CAD build for the part. Positions are in the model's coordinates, mm. Coordinates: 2 decimals unless noted, no trailing zeros. Loops run counter-clockwise (first coordinate to the right, second up) from the corner with the lowest first, then second, coordinate; pieces in that order, holes last. Notation, with made-up numbers: (-30.75, 18) -> (-22.75, 18) arc R8 cw to (-22.75, 31) -> close; hole circle Ø4 at (8.5, -4). An arc over 180 degrees is marked (long way). Answer as CSV lines item,"result". Start each with the question number.
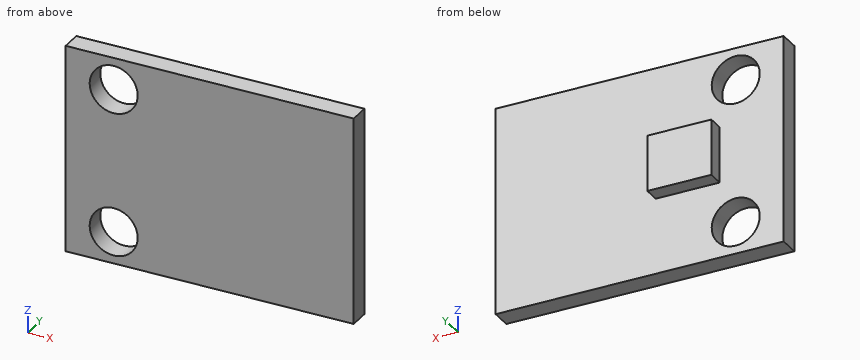
```python
from build123d import *

# Parameters (mm, degrees)
SKETCH1_W           = 18
SKETCH1_H           = 13
BOSS_EXTRUDE1_DEPTH = 1.27
CUT_EXTRUDE1_REACH  = 13.174
SKETCH2_R           = 1.5
CUT_EXTRUDE2_REACH  = 13.174
SKETCH3_R           = 1.5
SKETCH4_W           = 4
SKETCH4_H           = 3.5
BOSS_EXTRUDE2_DEPTH = 1


with BuildPart() as part:
    # Sketch1 → Boss-Extrude1 (new body)
    with BuildSketch(Plane(origin=(0, 0, 0), x_dir=(1, 0, 0), z_dir=(0, 1, 0))):
        Rectangle(SKETCH1_W, SKETCH1_H)
    extrude(amount=BOSS_EXTRUDE1_DEPTH)

    # Sketch2 → Cut-Extrude1 (cut, up to next)
    with BuildSketch(Plane(origin=(0, 1.27, 0), x_dir=(1, 0, 0), z_dir=(0, 1, 0)), mode=Mode.PRIVATE) as cut_extrude1_sk1:
        with Locations(Location((-6, 4.5, 0), (0, 0, 270))):
            Circle(SKETCH2_R)
    cut_extrude1_tool1 = extrude(cut_extrude1_sk1.sketch, amount=-CUT_EXTRUDE1_REACH, mode=Mode.PRIVATE) & part.part
    add(cut_extrude1_tool1.solids().sort_by_distance((-6, 1.27, -4.5))[0], mode=Mode.SUBTRACT)

    # Sketch3 → Cut-Extrude2 (cut, up to next)
    with BuildSketch(Plane(origin=(0, 1.27, 0), x_dir=(1, 0, 0), z_dir=(0, 1, 0)), mode=Mode.PRIVATE) as cut_extrude2_sk1:
        with Locations(Location((-6, -4.5, 0), (0, 0, 270))):
            Circle(SKETCH3_R)
    cut_extrude2_tool1 = extrude(cut_extrude2_sk1.sketch, amount=-CUT_EXTRUDE2_REACH, mode=Mode.PRIVATE) & part.part
    add(cut_extrude2_tool1.solids().sort_by_distance((-6, 1.27, 4.5))[0], mode=Mode.SUBTRACT)

    # Sketch4 → Boss-Extrude2 (add)
    with BuildSketch(Plane(origin=(0, 1.27, 0), x_dir=(1, 0, 0), z_dir=(0, 1, 0))):
        with Locations((-3, 0)):
            Rectangle(SKETCH4_W, SKETCH4_H)
    extrude(amount=BOSS_EXTRUDE2_DEPTH)


solid = part.part
```
Q1. Pin check, flat tips, straight feed: pin 1 Ø1.1 at (y, z) = (1.5, 0) entering from +X; pin 2 Ø2.5 at (x, z) = (-6, -4.5) entering from -Y; pin 3 Ø0.5 at (x, y) = (-3.5, 2) entering from -Z; pin 4 Ø4 at (x, z) = (5.5, 3.5) entering from +Y. Stop position of each tip, or through.
Q2. Saw through at B-B (x = -6). List the corners of the cut face in (y, z).
Q3. Saw through at D-D (z = 1.5). List the corners of the cut face in (x, y), and give its area (3 significant figures).
Q4. Saw through at C-C (y = 0.6). List the corners of the cut face in (x, z), and give its area (3 significant figures).
Q5. Saw through at A-A (z = 4.5). List the corners of the cut face in (x, y).
Q6. Probe probe 1 along X at (y, z) = (0.4, 4.5); probe 2 along Z at (x, y) = (-7, 0.9); probe 3 along Y at (x, z) = (2.5, 6.25). List the from-to ranges inside material, lowest first. Write a range as from..to.
Ans:
1,pin 1,"stops at x = 9"
1,pin 2,"passes through"
1,pin 3,"stops at z = -1.75"
1,pin 4,"stops at y = 1.27"
2,outline,"(0, -6.5) -> (1.27, -6.5) -> (1.27, -6) -> (0, -6) -> close; (0, -3) -> (1.27, -3) -> (1.27, 3) -> (0, 3) -> close; (0, 6) -> (1.27, 6) -> (1.27, 6.5) -> (0, 6.5) -> close"
3,outline,"(-9, 0) -> (9, 0) -> (9, 1.27) -> (-1, 1.27) -> (-1, 2.27) -> (-5, 2.27) -> (-5, 1.27) -> (-9, 1.27) -> close"
3,area,"26.9 mm²"
4,outline,"(-9, -6.5) -> (9, -6.5) -> (9, 6.5) -> (-9, 6.5) -> close; hole circle Ø3 at (-6, -4.5); hole circle Ø3 at (-6, 4.5)"
4,area,"220 mm²"
5,outline,"(-9, 0) -> (-7.5, 0) -> (-7.5, 1.27) -> (-9, 1.27) -> close; (-4.5, 0) -> (9, 0) -> (9, 1.27) -> (-4.5, 1.27) -> close"
6,probe 1,"x = -9..-7.5, -4.5..9"
6,probe 2,"z = -6.5..-5.62, -3.38..3.38, 5.62..6.5"
6,probe 3,"y = 0..1.27"
